```python
from build123d import *

# Parameters (mm, degrees)
SKETCH1_R           = 47.5
SKETCH1_R_2         = 34.5
BOSS_EXTRUDE1_DEPTH = 15
SKETCH2_R           = 2.25
CUT_EXTRUDE1_DEPTH  = 69.82949949
SKETCH3_R           = 4
CUT_EXTRUDE2_DEPTH  = 4.4
FILLET1_R           = 1
FILLET2_R           = 0.5


with BuildPart() as part:
    # Sketch1 → Boss-Extrude1 (new body)
    with BuildSketch(Plane(origin=(0, 0, 0), x_dir=(1, 0, 0), z_dir=(0, 1, 0))):
        with Locations(Location((0, 0, 0), (0, 0, 270))):
            Circle(SKETCH1_R)
        with Locations(Location((0, 0, 0), (0, 0, 270))):
            Circle(SKETCH1_R_2, mode=Mode.SUBTRACT)
    extrude(amount=BOSS_EXTRUDE1_DEPTH)

    # Sketch2 → Cut-Extrude1 (cut, through all)
    with BuildSketch(Plane(origin=(0, 15, 0), x_dir=(1, 0, 0), z_dir=(0, 1, 0))):
        with Locations(Location((0, 41.5, 0), (0, 0, 270))):
            Circle(SKETCH2_R)
        with Locations(Location((29.344931419, 29.344931419, 0), (0, 0, 270))):
            Circle(SKETCH2_R)
        with Locations(Location((41.5, 0, 0), (0, 0, 270))):
            Circle(SKETCH2_R)
        with Locations(Location((29.344931419, -29.344931419, 0), (0, 0, 270))):
            Circle(SKETCH2_R)
        with Locations(Location((0, -41.5, 0), (0, 0, 270))):
            Circle(SKETCH2_R)
        with Locations(Location((-29.344931419, -29.344931419, 0), (0, 0, 270))):
            Circle(SKETCH2_R)
        with Locations(Location((-41.5, 0, 0), (0, 0, 270))):
            Circle(SKETCH2_R)
        with Locations(Location((-29.344931419, 29.344931419, 0), (0, 0, 270))):
            Circle(SKETCH2_R)
    extrude(amount=-CUT_EXTRUDE1_DEPTH, mode=Mode.SUBTRACT)

    # Sketch3 → Cut-Extrude2 (cut)
    with BuildSketch(Plane(origin=(0, 15, 0), x_dir=(1, 0, 0), z_dir=(0, 1, 0))):
        with Locations(Location((0, 41.5, 0), (0, 0, 270))):
            Circle(SKETCH3_R)
        with Locations(Location((29.344931419, 29.344931419, 0), (0, 0, 270))):
            Circle(SKETCH3_R)
        with Locations(Location((41.5, 0, 0), (0, 0, 270))):
            Circle(SKETCH3_R)
        with Locations(Location((29.344931419, -29.344931419, 0), (0, 0, 270))):
            Circle(SKETCH3_R)
        with Locations(Location((0, -41.5, 0), (0, 0, 270))):
            Circle(SKETCH3_R)
        with Locations(Location((-29.344931419, -29.344931419, 0), (0, 0, 270))):
            Circle(SKETCH3_R)
        with Locations(Location((-41.5, 0, 0), (0, 0, 270))):
            Circle(SKETCH3_R)
        with Locations(Location((-29.344931419, 29.344931419, 0), (0, 0, 270))):
            Circle(SKETCH3_R)
    extrude(amount=-CUT_EXTRUDE2_DEPTH, mode=Mode.SUBTRACT)

    # Fillet1
    fillet1_edges = [part.edges().sort_by_distance(p)[0] for p in [
        (0, 0, -47.5),
        (0, 15, -47.5),
    ]]
    fillet(fillet1_edges, radius=FILLET1_R)

    # Fillet2
    fillet2_edges = [part.edges().sort_by_distance(p)[0] for p in [
        (0, 0, -34.5),
        (0, 15, -34.5),
    ]]
    fillet(fillet2_edges, radius=FILLET2_R)


solid = part.part
```
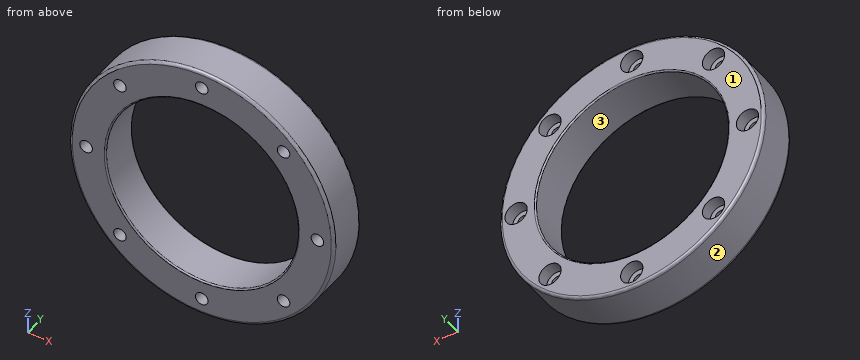
For this review, take the finished solid that the model builds, in its own axes (mm). Face numbers are marked on the shaded views. Coordinates: 2 decimals unless noted, no trailing zeros. Put each result on its own line as item: value.
Q1. Take a section at A-A, the plane z = 0. Count the separate pieces of the cut face and the enclosed holes in it, then the cut area to 3 significant figures.
From the geometry:
separate pieces: 4
enclosed holes: 0
area: 223 mm2
Q2. The part is to be moulded in two halves that separate along X. For the marked faces 1, 2 and 3, say which applies: +X half, -X half, draft (parallel to the pull), parting line (faces both ways), or undercut.
From the geometry:
face 1: draft
face 2: parting line
face 3: undercut
Q3. Clearance check with flat-ended pins moving along their axes: pin 1 Ø3.5 at (x, z) = (0, 41.5) entering from -Y; pin 2 Ø6 at (x, z) = (29.34, -29.34) entering from +Y; pin 3 Ø8 at (x, y) = (8.5, 4.5) entering from +Z; pin 4 Ø1 at (x, y) = (10, 4.5) entering from +Z. State where each tip first meets the part, or that it passes through.
From the geometry:
pin 1: passes through
pin 2: stops at y = 10.6
pin 3: stops at z = 47.29
pin 4: stops at z = 46.54
Q4. Wall thickness on L1, parallel to Z at x = -29.5, y = 7; L2, parallel to Z at x = 0.5, y = 2.75; L3, parallel to X at y = 8, z = 28: over which ranges is each line inside the solid? List them lowest first.
From the geometry:
L1: z = -37.23 to -31.59, -27.1 to -17.89, 17.89 to 27.1, 31.59 to 37.23
L2: z = -47.5 to -43.69, -39.31 to -34.5, 34.5 to 39.31, 43.69 to 47.5
L3: x = -38.37 to -31.15, -27.54 to -20.16, 20.16 to 27.54, 31.15 to 38.37
